Input: dimensioned drawing with shaded views. Units: mm. Origin: part minimum x, y, z. A direction names the side the tool comes from. Coordinates: 2 decimals unless noted, no trailing zeros. Loops run counter-clockwise (first coordinate to the right, second up) from the corner with the lowest first, then second, coordinate; pieces in that order, holes last.
Item 1: Reachability of the marked faces 1 and 2 from +Z, -Z, +X, -X, +Y, -Y: full face, straight path, thin tool, end or side. Return the list, or none.
Item 2: Section C-C on z = 35. Return loops of the section in (x, y), and give its area (3 significant figures).
Item 3: Ray query, line 1 along Z through (x, y) = (10.75, 18.25); line 2 along Z through (x, y) = (15, 20.5); line 3 along Y through (x, z) = (7.75, 43.5). Return the intervals inside material, ascending.
Item 4: Contact query for flat-ended pins moving along their axis: P1, Ø3, axis at y = 4.5, z = 17.5, coming from the -X side; P2, Ø8, axis at x = 11, z = 16, coming from the +Y side; P3, Ø6, axis at x = 4, z = 29, coming from the +Y side. Output: stop coordinate, or through.
Item 5: Section A-A on x = 11.5. Return loops of the section in (y, z), and give its area (3 significant figures).
Item 6: Section D-D on x = 19.5. Return loops of the section in (y, z).
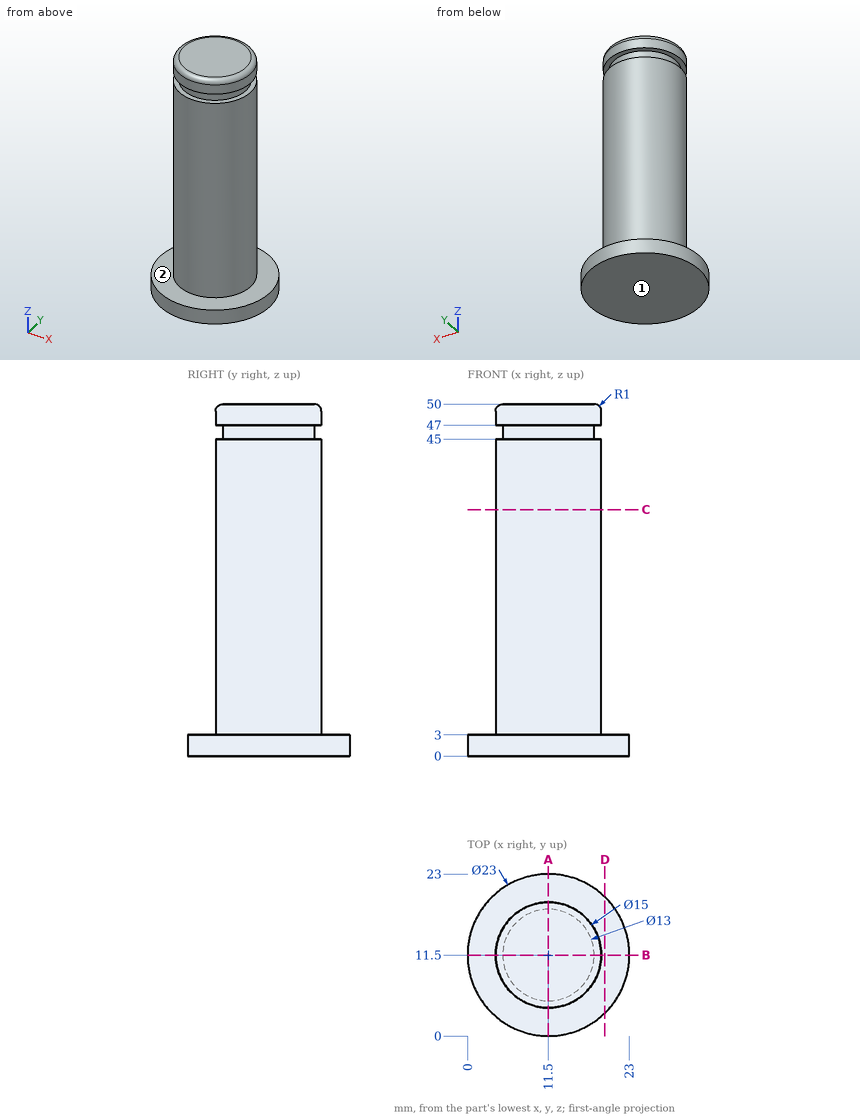
Results found:
1. face 1: -Z, +X, -X, +Y, -Y
1. face 2: +Z
2. outline: circle Ø15 at (11.5, 11.5)
2. area: 177 mm2
3. line 1: z = 0 to 45, 47 to 49.96
3. line 2: z = 0 to 3
3. line 3: y = 5 to 18
4. P1: stops at x = 6.4
4. P2: stops at y = 19
4. P3: stops at y = 17.5
5. outline: (0, 0) - (23, 0) - (23, 3) - (19, 3) - (19, 45) - (18, 45) - (18, 47) - (19, 47) - (19, 49) arc R1 ccw to (18, 50) - (5, 50) arc R1 ccw to (4, 49) - (4, 47) - (5, 47) - (5, 45) - (4, 45) - (4, 3) - (0, 3) - close
5. area: 770 mm2
6. outline: (3.24, 0) - (19.76, 0) - (19.76, 3) - (3.24, 3) - close
